Autodesk Inventor part; units mm, degrees
ref_plane "YZ Plane" through (0, 0, 0) normal (1, 0, 0) x (0, 1, 0)
ref_plane "XZ Plane" through (0, 0, 0) normal (0, 1, 0) x (-1, 0, 0)
ref_plane "XY Plane" through (0, 0, 0) normal (0, 0, 1) x (1, 0, 0)
sketch "Sketch1" plane through (0, 0, 0) normal (0, 1, 0) x (-1, 0, 0)
  line L0 (0, -7.9375) -> (0, 7.9375) construction
  line L1 (17.4625, -7.9375) -> (17.4625, 7.9375)
  line L2 (-17.4625, 7.9375) -> (-17.4625, -7.9375)
  arc A0 (-17.4625, -7.9375) -> (17.4625, -7.9375) centre (0, -7.9375) ccw
  arc A1 (17.4625, 7.9375) -> (-17.4625, 7.9375) centre (0, 7.9375) ccw
  line L3 (14.2875, 7.9375) -> (14.2875, -7.9375)
  arc A2 (-14.2875, -7.9375) -> (14.2875, -7.9375) centre (0, -7.9375) ccw
  line L4 (-14.2875, -7.9375) -> (-14.2875, 7.9375)
  arc A3 (14.2875, 7.9375) -> (-14.2875, 7.9375) centre (0, 7.9375) ccw
  point P0 (0, 0)
  point P1 (0, 25.4)
  point P2 (0, -25.4)
  dimension "d1" = 34.925
  dimension "d2" = 3.175
  dimension "d3" = 50.8
extrude "Extrusion1" add sketch "Sketch1" along normal mid plane 25.4
sketch "Sketch2" plane through (17.4625, -12.7, -7.9375) normal (1, 0, 0) x (0, 0, -1)
  line L0 (0, 0) -> (0, 25.4) construction
  line L1 (-15.875, 25.4) -> (0, 25.4) construction
  line L2 (-15.875, 0) -> (-15.875, 25.4) construction
  line L3 (0, 0) -> (-15.875, 0) construction
  line L4 (-15.875, 0) -> (-15.875, 25.4) construction
  line L5 (-15.875, 25.4) -> (-15.875, 25.4) construction
  line L6 (-15.875, 25.4) -> (-15.875, 0) construction
  line L7 (-15.875, 0) -> (-15.875, 0) construction
  line L8 (0, 0) -> (0, 25.4) construction
  line L9 (0, 25.4) -> (0, 25.4) construction
  line L10 (0, 0) -> (0, 25.4) construction
  line L11 (0, 0) -> (0, 0) construction
  line L12 (-15.875, 25.4) -> (-33.3375, 25.4) construction
  line L13 (17.4625, 0) -> (17.4625, 25.4) construction
  line L14 (-33.3375, 25.4) -> (17.4625, 25.4)
  line L15 (17.4625, 25.4) -> (17.4625, 0)
  line L16 (17.4625, 0) -> (-33.3375, 0)
  line L17 (-33.3375, 0) -> (-33.3375, 25.4)
  line L18 (0, 0) -> (-15.875, 0) construction
  circle A0 centre (-26.9875, 12.7) radius 3.375
  circle A1 centre (11.1125, 12.7) radius 3.375
  line L19 (-26.9875, 12.7) -> (11.1125, 12.7) construction
  point P0 (-7.9375, 12.7)
  point P1 (-7.9375, 12.7)
  dimension "d6" = 6.75
  dimension "d7" = 38.1
extrude "Extrusion2" add sketch "Sketch2" against normal up to next
extrude "Extrusion3" cut sketch "Sketch1" along normal mid plane 25.4 contours L3 A2 L4 A3
chamfer "Chamfer1" distance 1.5875 angle 45 4 edges at (-14.2875, 12.7, 0) (0, 12.7, -22.225) (14.2875, 12.7, 0) (0, 12.7, 22.225)
properties part number "WL-005" material "Aluminum 6061"
Input: part model. Units: mm. Frame: model coordinates. A direction names the side the tool comes from. Round coordinates to 2 decimals unless told otherwise and drop trailing zeros. Order: outer loops, then holes, each group sorted by start corner. A loop starts at its lowest first (then second) coordinate and runs counter-clockwise, first axis right, second up. Notation, with made-up numbers: (89.25, 63.25) - (134.25, 63.25) arc R29 ccw to (134.25, 99.25) - close; hole circle Ø10 at (-37.5, -6.75). An arc over 180 degrees is marked (long way). Answer as a JSON object with one key per item and string values. Group by question number.
(1) Material intervals for probe 1 along Y at (x, z) = (15, 19.05) (3 decimals); probe 2 along Z at (x, y) = (16.25, 0) (3 decimals); probe 3 along X at (y, z) = (11, -6.5), sorted ascending. Write a range as from..to.
(2) Pin query (flat end, axial travel): P1, Ø1.5, axis at x = -7, y = 4.5, coming from the +Z side; P2, Ø4, axis at x = -12.5, z = -1, coming from the +Y side (3 decimals); P3, Ø6, axis at y = 0, z = -19.05, coming from the -X side. Return the tip coordinate at first contact, or that it passes through.
(3) Cut plane C-C (x = 13.5). Count the separate pieces of the cut face and the enclosed holes in it, then the cut area to 3 significant figures.
(4) Cut plane A-A (z = -6.5). Return loops of the section in (x, y) (1 decimal), then the cut area to 3 significant figures.
(5) Draft query along Z for faces 1 (the face through (9, 0, -25.4)), 2 (the face through (16, -12.7, 2)), 3 (the face through (13.101, -0.047, -19.483)). Return one class per face: released by +Z, released by -Z, zero draft, split by the parting line, or undercut.
(6) Cut plane B-B (y = 0). Return loops of the section in (x, z) (1 decimal), then the cut area to 3 significant figures.
(7) Reachability of faces 4 (the face through (14.52, 0.15, 22.42)), 5 (the face through (0.32, 11.39, -22.5)), 6 (the face through (-17.462, 0, 0)), 7 (the face through (0.31, -0.96, 22.22)), 8 (the face through (17, 12.7, 2)) from +Z, -Z, +X, -X, +Y, -Y: full face, straight path, thin tool, end or side. Return the list, or none.
Here are the results:
{
 "1": {"probe 1": "y = -12.7..-3.375, 3.375..12.7", "probe 2": "z = -25.4..-22.425, -15.675..15.675, 22.425..25.4", "probe 3": "x = -17.46..-14.29, 14.29..17.46"},
 "2": {"P1": "stops at z = 24.24", "P2": "stops at y = 11.325", "P3": "stops at x = -15.46"},
 "3": {"separate pieces": "2", "enclosed holes": "2", "area": "607 mm^2"},
 "4": {"outline": "(-17.5, -12.7) - (-14.3, -12.7) - (-14.3, 11.1) - (-15.9, 12.7) - (-17.5, 12.7) - close; (14.3, -12.7) - (17.5, -12.7) - (17.5, 12.7) - (15.9, 12.7) - (14.3, 11.1) - close", "area": "159 mm^2"},
 "5": {"face 1": "released by -Z", "face 2": "zero draft", "face 3": "undercut"},
 "6": {"outline": "(-17.5, -7.9) arc R17.5 ccw to (0, -25.4) - (17.5, -25.4) - (17.5, -22.4) - (9.7, -22.4) arc R17.5 ccw to (15.7, -15.7) - (17.5, -15.7) - (17.5, 15.7) - (15.7, 15.7) arc R17.5 ccw to (9.7, 22.4) - (17.5, 22.4) - (17.5, 25.4) - (0, 25.4) arc R17.5 ccw to (-17.5, 7.9) - close; hole (-14.3, -7.9) arc R14.3 ccw to (14.3, -7.9) - (14.3, 7.9) arc R14.3 ccw to (-14.3, 7.9) - close", "area": "491 mm^2"},
 "7": {"face 4": "+X", "face 5": "+Y", "face 6": "+Z, -Z, -X, +Y, -Y", "face 7": "+Y, -Y", "face 8": "+Z, -Z, +X, -X, +Y"}
}
